Read the model definition and answer for the solid it produces. Units are mm, in the model's axes. A direction names the side the tool comes from. Coordinates: 2 decimals unless noted, no trailing zeros. Loops run counter-clockwise (first coordinate to the right, second up) from the corner with the lowest first, then second, coordinate; pieces in that order, holes last. Notation, with made-up numbers: (49, 9) -> (103, 9) arc R30 cw to (103, 47) -> close; hole circle Ø10 at (-35.5, 69.5). An arc over 180 degrees is marked (long way). Answer as a JSON object with one key per item and string values. Group by question number.
Q1. The part is cut by section A-A on y = 12.15. Write down the section's boundary in (x, z), and give its area (3 significant figures).
Q2. Straight lines are drawn through the part: line 1 along Z through (x, y) = (-3.25, 3); line 2 along Y through (x, z) = (-0.4, 23.1); line 3 along Z through (x, y) = (-8.7, 5). For each, find the intervals that lie inside material, in ascending order. Write a range as [from, to].
Q3. Each of these flat-tipped pins is pushed along its axis until it touches: P1, Ø1.4, axis at x = -3, z = 10.5, coming from the -Y side; P2, Ø1.5, axis at y = -10.5, z = 13.5, coming from the +X side; P3, Ø1.4, axis at y = 2, z = 0.5, coming from the -X side; P4, Ø1.4, axis at x = -2.5, z = 10, coming from the +Y side. Where does it stop, or does it pass through?
Q4. The part is cut by section D-D on x = -8.5. Write down the section's boundary in (y, z), and give its area (3 significant figures).
Q5. Determine the mould class of faces 1 (the cylindrical face through (-1.201, 0.091, 8.785)), 2 (the cylindrical face through (-0.76, -13.76, 23.24)), 3 (the flat face through (0, 0, 22.5)) for opening direction X: released by +X, released by -X, zero draft, split by the parting line, or undercut.
Q6. For faces 4 (the flat face through (-4, -10, 0)), 5 (the flat face through (-2, 6.5, 11)), 6 (the flat face through (-4.6, 8.8, 5.25)), 7 (the flat face through (-3, 0, 0)), determine the directions among +Z, -Z, +X, -X, +Y, -Y from which every point of the face is accessible in a straight line to the end or side of a thin tool.
Q7. The part is cut by section B-B on x = -3. Write down the section's boundary in (y, z).
Q8. The part is cut by section C-C on y = -12.15. Write down the section's boundary in (x, z).
from build123d import *

# Parameters (mm, degrees)
BOSS_EXTRUDE1_DEPTH      = 5
BOSS_EXTRUDE1_DEPTH_BACK = 5
SKETCH2_W                = 3.6
SKETCH2_H                = 10
BOSS_EXTRUDE2_DEPTH      = 1
SKETCH3_W                = 1
SKETCH3_H                = 10
BOSS_EXTRUDE3_DEPTH      = 1.5
SKETCH4_W                = 1.5
SKETCH4_H                = 30
SKETCH4_W_2              = 6.5
SKETCH4_R                = 1.65
BOSS_EXTRUDE4_DEPTH      = 1.5
FILLET1_R                = 0.3
SKETCH5_W                = 4
SKETCH5_H                = 13
BOSS_EXTRUDE5_DEPTH      = 2.7
CUT_EXTRUDE1_DEPTH       = 30.038767191
BOSS_EXTRUDE6_START      = -1.5
BOSS_EXTRUDE6_DEPTH      = 5
CUT_EXTRUDE2_START       = -3
SKETCH8_W                = 2.5
SKETCH8_H                = 6
CUT_EXTRUDE2_DEPTH       = 3
FILLET2_R                = 3
FILLET3_R                = 1
FILLET4_R                = 1


with BuildPart() as part:
    # Sketch1 → Boss-Extrude1 (new, two sides: drawn at the far end of the back side and taken through both)
    with BuildSketch(Plane(origin=(0, 0, 0), x_dir=(1, 0, 0), z_dir=(0, 1, 0)).offset(-BOSS_EXTRUDE1_DEPTH_BACK)):
        Polygon((0, 0), (-2.2, 0), (-2.2, -1.270170592), align=None)
    extrude(amount=BOSS_EXTRUDE1_DEPTH + BOSS_EXTRUDE1_DEPTH_BACK)

    # Sketch2 → Boss-Extrude2 (add)
    with BuildSketch(Plane(origin=(0, 0, 0), x_dir=(-1, 0, 0), z_dir=(0, 0, -1))):
        with Locations((1.8, 0)):
            Rectangle(SKETCH2_W, SKETCH2_H)
    extrude(amount=BOSS_EXTRUDE2_DEPTH)

    # Sketch3 → Boss-Extrude3 (add)
    with BuildSketch(Plane.ZY.offset(3.6)):
        Polygon((0, -5), (0, -15), (22.5, -15), (22.5, 15), (0, 15), (0, 5), align=None)
        with Locations((-0.5, 0)):
            Rectangle(SKETCH3_W, SKETCH3_H)
    extrude(amount=BOSS_EXTRUDE3_DEPTH)

    # Sketch4 → Boss-Extrude4 (add)
    # profile 1 of 2: a face of its own
    with BuildSketch(Plane.XY.offset(22.5)):
        with Locations((-4.35, 0)):
            Rectangle(SKETCH4_W, SKETCH4_H)
    # profile 2 of 2: a face of its own
    with BuildSketch(Plane.XY.offset(22.5)):
        with Locations((-0.35, 0)):
            Rectangle(SKETCH4_W_2, SKETCH4_H)
        with Locations((-0.4, -12.15)):
            Circle(SKETCH4_R, mode=Mode.SUBTRACT)
        with Locations((-0.4, 12.15)):
            Circle(SKETCH4_R, mode=Mode.SUBTRACT)
    extrude(amount=BOSS_EXTRUDE4_DEPTH)

    # Fillet1
    fillet1_edges = [part.edges().sort_by_distance(p)[0] for p in [
        (0, 0, -1),
        (-5.1, 10, 0),
        (-5.1, -10, 0),
        (-5.1, 0, -1),
        (2.9, 0, 24),
        (-5.1, 0, 24),
    ]]
    fillet(fillet1_edges, radius=FILLET1_R)

    # Sketch5 → Boss-Extrude5 (add)
    with BuildSketch(Plane(origin=(-3.6, 0, 0), x_dir=(0, 0, -1), z_dir=(1, 0, 0))):
        with Locations((-10.5, 0)):
            Rectangle(SKETCH5_W, SKETCH5_H)
    extrude(amount=BOSS_EXTRUDE5_DEPTH)

    # Sketch7 → Cut-Extrude1 (cut, through all)
    with BuildSketch(Plane(origin=(-3.6, 0, 0), x_dir=(0, 0, -1), z_dir=(1, 0, 0))):
        with BuildLine():
            Line((-5.25, 6.299038106), (-5.25, 15))
            Line((-5.25, 15), (-6.75, 15))
            Line((-6.75, 15), (-6.75, 6.299038106))
            ThreePointArc((-6.75, 6.299038106), (-6, 3.5), (-5.25, 6.299038106))
        make_face()
    extrude(amount=-CUT_EXTRUDE1_DEPTH, mode=Mode.SUBTRACT)

    # Sketch7<3> → Boss-Extrude6 (add)
    with BuildSketch(Plane(origin=(-3.6, 0, 0), x_dir=(0, 0, -1), z_dir=(1, 0, 0)).offset(BOSS_EXTRUDE6_START)):
        with BuildLine():
            Line((-6.75, 6.299038106), (-6.75, 7.90473751))
            ThreePointArc((-6.75, 7.90473751), (-7.837117307, 2.628291755), (-3, 5))
            ThreePointArc((-3, 5), (-3.628291755, 6.837117307), (-5.25, 7.90473751))
            Line((-5.25, 7.90473751), (-5.25, 6.299038106))
            ThreePointArc((-5.25, 6.299038106), (-4.700961894, 5.75), (-4.5, 5))
            ThreePointArc((-4.5, 5), (-6.75, 3.700961894), (-6.75, 6.299038106))
        make_face()
    extrude(amount=-BOSS_EXTRUDE6_DEPTH)

    # Sketch8 → Cut-Extrude2 (cut)
    with BuildSketch(Plane(origin=(0, 2, 0), x_dir=(-1, 0, 0), z_dir=(0, -1, 0)).offset(CUT_EXTRUDE2_START)):
        with Locations((8.85, -6)):
            Rectangle(SKETCH8_W, SKETCH8_H)
    extrude(amount=CUT_EXTRUDE2_DEPTH, mode=Mode.SUBTRACT)

    # Fillet2
    # the kernel refuses this fillet: 3 mm, written as the material it adds along each edge
    with BuildSketch(Plane(origin=(-7.6, 5, -4.395099729), x_dir=(-1, 0, 0), z_dir=(0, 0, 1))) as fillet2_piece_1_section:
        with BuildLine():
            CenterArc((3, 2.958039892), FILLET2_R, 180, 80.405931773)
            Line((0, 2.958039892), (0, 0))
            Line((0, 0), (2.5, 0))
        make_face()
    fillet2_piece_1 = extrude(amount=16.290199458, mode=Mode.PRIVATE)
    fillet2_piece_1 = fillet2_piece_1 & Plane(origin=(-7.6, 5, 6), x_dir=(0, 0.9682458365518564, 0.2499999999999917), z_dir=(1, 0, 0)) * Cylinder(3, 45, mode=Mode.PRIVATE)
    fillet2_piece_1 = fillet2_piece_1 - Plane(origin=(-7.6, 5, 6), x_dir=(0, 0.8660254037844379, -0.5000000000000012), z_dir=(1, 0, 0)) * Cylinder(1.5, 45, mode=Mode.PRIVATE)
    add(fillet2_piece_1)

    # Fillet3
    fillet3_edges = [part.edges().sort_by_distance(p)[0] for p in [
        (-5.1, 2.628291755, 7.837117307),
    ]]
    fillet(fillet3_edges, radius=FILLET3_R)

    # Fillet4
    fillet4_edges = [part.edges().sort_by_distance(p)[0] for p in [
        (-0.9, 0, 8.5),
        (-0.9, 0, 12.5),
    ]]
    fillet(fillet4_edges, radius=FILLET4_R)


solid = part.part
Final values:
{
 "1": {"outline": "(-5.1, 0.3) arc R0.3 ccw to (-4.8, 0) -> (-3.6, 0) -> (-3.6, 5.25) -> (-5.1, 5.25) -> close; (-5.1, 6.75) -> (-3.6, 6.75) -> (-3.6, 22.5) -> (-2.05, 22.5) -> (-2.05, 24) -> (-4.8, 24) arc R0.3 ccw to (-5.1, 23.7) -> close; (1.25, 22.5) -> (2.9, 22.5) -> (2.9, 23.7) arc R0.3 ccw to (2.6, 24) -> (1.25, 24) -> close", "area": "38.5 mm2"},
 "2": {"line 1": "z = [-1, 0], [8.5, 12.5], [22.5, 24]", "line 2": "y = [-15, -13.8], [-10.5, 10.5], [13.8, 15]", "line 3": "z = [3, 4.5], [7.5, 9]"},
 "3": {"P1": "stops at y = -15", "P2": "stops at x = -3.6", "P3": "stops at x = -5.1", "P4": "stops at y = 6.5"},
 "4": {"outline": "(4.18, 3.11) arc R3 ccw to (7.9, 5.25) -> (6.3, 5.25) arc R1.5 cw to (4.18, 4.74) -> close; (4.18, 7.26) arc R1.5 cw to (6.3, 6.75) -> (7.9, 6.75) arc R3 ccw to (4.18, 8.89) -> close", "area": "10.8 mm2"},
 "5": {"face 1": "released by +X", "face 2": "undercut", "face 3": "zero draft"},
 "6": {"face 4": "-Z, +X, -X, -Y", "face 5": "-Z, +X, +Y", "face 6": "+X, -X, +Y", "face 7": "+Y, -Y"},
 "7": {"outline": "(-15, 22.5) -> (15, 22.5) -> (15, 24) -> (-15, 24) -> close; (-6.5, 8.5) -> (6.5, 8.5) -> (6.5, 12.5) -> (-6.5, 12.5) -> close; (-5, -1) -> (5, -1) -> (5, 0) -> (-5, 0) -> close"},
 "8": {"outline": "(-5.1, 0.3) arc R0.3 ccw to (-4.8, 0) -> (-3.6, 0) -> (-3.6, 22.5) -> (-2.05, 22.5) -> (-2.05, 24) -> (-4.8, 24) arc R0.3 ccw to (-5.1, 23.7) -> close; (1.25, 22.5) -> (2.9, 22.5) -> (2.9, 23.7) arc R0.3 ccw to (2.6, 24) -> (1.25, 24) -> close"}
}
